```python
from build123d import *

# Parameters (mm, degrees)
SKETCH1_R             = 80
SKETCH1_R_2           = 6
BOSS_EXTRUDE1_DEPTH   = 13
SKETCH2_R             = 65
CUT_EXTRUDE1_DEPTH    = 8
MIRROR1_START         = -13
MIRROR1_OUTLINE_R     = 65
MIRROR1_OUTLINE_R_2   = 6
MIRROR1_DEPTH         = 8
MIRROR1_START_2       = -3
MIRROR1_2_OUTLINE_R   = 65
MIRROR1_2_OUTLINE_R_2 = 6
MIRROR1_2_DEPTH       = 8
SKETCH3_R             = 13
SKETCH3_R_2           = 6
BOSS_EXTRUDE2_DEPTH   = 18
CHAMFER1_SIZE         = 1
CUT_EXTRUDE2_DEPTH    = 116.06954419
CIRPATTERN1_COUNT     = 10


# Read off the part's stored shape, not the designer's step: Mirror1
with BuildPart() as part:
    # Sketch1 → Boss-Extrude1 (new, symmetric)
    with BuildSketch(Plane.XY):
        with Locations(Location((0, 0, 0), (0, 0, 180))):
            Circle(SKETCH1_R)
        with Locations(Location((0, 0, 0), (0, 0, 180))):
            Circle(SKETCH1_R_2, mode=Mode.SUBTRACT)
    extrude(amount=BOSS_EXTRUDE1_DEPTH, both=True)

    # Sketch2 → Cut-Extrude1 (cut)
    with BuildSketch(Plane.XY.offset(13)):
        Circle(SKETCH2_R)
    extrude(amount=-CUT_EXTRUDE1_DEPTH, mode=Mode.SUBTRACT)

    # Mirror1 outline → Mirror1 (cut)
    with BuildSketch(Plane.XY.offset(MIRROR1_START)):
        Circle(MIRROR1_OUTLINE_R)
        Circle(MIRROR1_OUTLINE_R_2, mode=Mode.SUBTRACT)
    extrude(amount=MIRROR1_DEPTH, mode=Mode.SUBTRACT)

    # Mirror1 2 outline → Mirror1 2 (cut)
    with BuildSketch(Plane.XY.offset(MIRROR1_START_2)):
        Circle(MIRROR1_2_OUTLINE_R)
        Circle(MIRROR1_2_OUTLINE_R_2, mode=Mode.SUBTRACT)
    extrude(amount=MIRROR1_2_DEPTH, mode=Mode.SUBTRACT)

    # Sketch3 → Boss-Extrude2 (add, symmetric)
    with BuildSketch(Plane.XY):
        with Locations(Location((0, 0, 0), (0, 0, 180))):
            Circle(SKETCH3_R)
        with Locations(Location((0, 0, 0), (0, 0, 180))):
            Circle(SKETCH3_R_2, mode=Mode.SUBTRACT)
    extrude(amount=BOSS_EXTRUDE2_DEPTH, both=True)

    # Chamfer1
    chamfer1_edges = [part.edges().sort_by_distance(p)[0] for p in [
        (-65, 0, 13),
        (-65, 0, -13),
        (80, 0, -13),
        (80, 0, 13),
    ]]
    chamfer(chamfer1_edges, length=CHAMFER1_SIZE)

    # Sketch4 → Cut-Extrude2 (cut, through all)
    with BuildSketch(Plane.XY.offset(-3)):
        with BuildLine():
            Line((0, 19.397164741), (0, 54.772255751))
            ThreePointArc((0, 54.772255751), (-1.629000688, 58.46500048), (-5.454545455, 59.751551728))
            ThreePointArc((-5.454545455, 59.751551728), (-15.529142706, 57.955549577), (-25.152000934, 54.473634439))
            ThreePointArc((-25.152000934, 54.473634439), (-27.821744262, 51.446675992), (-27.386127875, 47.434164903))
            Line((-27.386127875, 47.434164903), (-9.698582371, 16.798437427))
            ThreePointArc((-9.698582371, 16.798437427), (-8.582686936, 15.895715021), (-7.149451403, 15.972956666))
            ThreePointArc((-7.149451403, 15.972956666), (-4.529333289, 16.90370196), (-1.794871795, 17.407711947))
            ThreePointArc((-1.794871795, 17.407711947), (-0.515032591, 18.057436487), (0, 19.397164741))
        make_face()
    cut_extrude2 = extrude(amount=-CUT_EXTRUDE2_DEPTH, mode=Mode.SUBTRACT)

    # CirPattern1: Cut-Extrude2 ×10 about axis
    cirpattern1_axis = Axis((0, 0, 0), (0, 0, 1))
    for i in range(1, CIRPATTERN1_COUNT):
        add(cut_extrude2.rotate(cirpattern1_axis, i * 360 / CIRPATTERN1_COUNT), mode=Mode.SUBTRACT)


solid = part.part
```
Geometry: final body of the model. Coordinates: model frame, mm. A direction names the side the tool comes from. Coordinates: 2 decimals unless noted, no trailing zeros. Order: outer loops, then holes, each group sorted by start corner. A loop starts at its lowest first (then second) coordinate and runs counter-clockwise, first axis right, second up. Notation, with made-up numbers: (-9, -2.75) - (3, -2.75) arc R17 cw to (3, 14.25) - close; hole circle Ø3 at (-40, 20.5). An arc over 180 degrees is marked (long way). Return JSON: item names as keys, results as strings. Group by question number.
1. Cut plane A-A (z = 9). Output: boundary loops of the cut face in (x, y), plus the area to 3 significant figures.
2. Pin query (flat end, axial travel): pin 1 (3 mm diameter, centred on x = -17.5, y = -22.5, fed in from +Z); pin 2 (10 mm diameter, centred on x = -59, z = 7.5, fed in from -Y); pin 3 (8 mm diameter, centred on x = 28, z = 12.5, fed in from +Y). Return the tip coordinate at first contact, or that it passes through.
3. Set-up query: faces 1 (the face through (-21.64, -55.96, -3.99)), 2 (the face through (62, 19.52, -8.55)), 3 (the face through (10.316, 7.91, 7.647)). Return all of +Z, -Z, +X, -X, +Y, -Y with unobstructed straight access to the full face (end or side cutting, diameter ignored); none if empty.
4. Cut plane B-B (y = 0). Count the separate pieces of the cut face and the enclosed holes in it, plus the area to 3 significant figures.
5. Material intervals for line 1 along Y through (x, z) = (0, 4); line 2 along Y through (x, z) = (1, -8); line 3 along Y through (x, z) = (8, 6.5), sorted ascending. Write a range as [from, to].
Resolved:
{
 "1": {"outline": "circle Ø160 at (0, 0); circle Ø26 at (0, 0); hole circle Ø130 at (0, 0); hole circle Ø12 at (0, 0)", "area": "7,250 mm²"},
 "2": {"pin 1": "stops at z = -3", "pin 2": "stops at y = -59.03", "pin 3": "stops at y = 76.31"},
 "3": {"face 1": "+Z, -Z", "face 2": "-Z", "face 3": "+Z"},
 "4": {"separate pieces": "4", "enclosed holes": "0", "area": "1,320 mm²"},
 "5": {"line 1": "y = [-80, -65], [-13, -6], [6, 13], [65, 80]", "line 2": "y = [-79.99, -64.99], [-12.96, -5.92], [5.92, 12.96], [64.99, 79.99]", "line 3": "y = [-79.6, -64.51], [-10.25, 10.25], [64.51, 79.6]"}
}
